from build123d import *

# Parameters (mm, degrees)
F0_W      = 15
F0_H      = 15
F1_DEPTH  = 25
F2_W      = 15
F2_H      = 15
F3_DEPTH  = 25
F4_DEPTH  = 10
F5_W      = 15
F5_H      = 15
F6_DEPTH  = 25
F7_W      = 5
F7_H      = 13
F8_DEPTH  = 25
F9_W      = 13
F9_H      = 5
F10_DEPTH = 20
F11_W     = 5
F11_H     = 13
F12_DEPTH = 25
F13_W     = 5
F13_H     = 5.5
F13_H_2   = 2.5
F14_DEPTH = 20


with BuildPart() as f1:
    # F0 (on Top) → F1 (new body)
    with BuildSketch(Plane.XY):
        with Locations((7.5, -7.5)):
            Rectangle(F0_W, F0_H)
    extrude(amount=F1_DEPTH)

    # F2 (on face) → F3 (join)
    with BuildSketch(Plane.XZ.offset(15)):
        with Locations((7.5, 7.5)):
            Rectangle(F2_W, F2_H)
    extrude(amount=F3_DEPTH)

    # F4 (add): a face of the model
    f4_faces = [f1.faces().sort_by_distance(p)[0] for p in [
        (7.5, -7.5, 25),
    ]]
    extrude(f4_faces, amount=F4_DEPTH)

    # F5 (on face) → F6 (join)
    with BuildSketch(Plane(origin=(0, 0, 0), x_dir=(0, -1, 0), z_dir=(-1, 0, 0))):
        with Locations((7.5, 7.5)):
            Rectangle(F5_W, F5_H)
    extrude(amount=F6_DEPTH)

    # F7 (on face) → F8 (cut, through all)
    with BuildSketch(Plane(origin=(-25, 0, 0), x_dir=(0, -1, 0), z_dir=(-1, 0, 0))):
        with Locations((10, 8.5)):
            Rectangle(F7_W, F7_H)
    extrude(amount=-F8_DEPTH, mode=Mode.SUBTRACT)

    # F9 (on face) → F10 (cut, through all)
    with BuildSketch(Plane.XY.offset(35)):
        with Locations((6.5, -10)):
            Rectangle(F9_W, F9_H)
    extrude(amount=-F10_DEPTH, mode=Mode.SUBTRACT)

    # F11 (on face) → F12 (cut, through all)
    with BuildSketch(Plane.XZ.offset(40)):
        with Locations((5, 8.5)):
            Rectangle(F11_W, F11_H)
    extrude(amount=-F12_DEPTH, mode=Mode.SUBTRACT)

    # F13 (on face) → F14 (cut, through all)
    with BuildSketch(Plane.XY.offset(35)):
        with Locations((5, -4.75)):
            Rectangle(F13_W, F13_H)
        with Locations((5, -13.75)):
            Rectangle(F13_W, F13_H_2)
    extrude(amount=-F14_DEPTH, mode=Mode.SUBTRACT)


solid = f1.part
Can you work these out from the model? Positions are in its coordinate system, mm. A direction names the side the tool comes from. Coordinates: 2 decimals unless noted, no trailing zeros. Write each loop counter-clockwise with the first axis right and the second up, starting at its lowest first coordinate (ties: lowest second). Pieces come first, ordered by that corner, then holes. Notation, with made-up numbers: M -30,-6 L -11,-6 A22 ccw -11,8 Z; hole C -36.5,27 d4. An arc over 180 degrees is marked long. Use one line per item in the form item = value.
Q1. For faces 1 (the flat face through (-12, -4, 15)), 2 (the flat face through (11, -27, 15)), 3 (the flat face through (-13, -10, 2)), 4 (the flat face through (5, -2, 25)), which set-ups out of +Z, -Z, +X, -X, +Y, -Y let a thin tool reach every point of the face, with its end or its side?
Model answer:
face_1 = +Z, -X, +Y, -Y
face_2 = +Z, +X, -X, -Y
face_3 = +Z, -X
face_4 = +Z, -Y
Q2. If we section it at B-B (x = 6): Write out the boundary of the cut face in (y, z).
Model answer:
outline = M -40,0 L 0,0 L 0,35 L -2,35 L -2,15 L -15,15 L -15,2 L -40,2 Z
Q3. If we section it at C-C (y = -18): Write out the boundary of the cut face in (x, z), then the cut area to 3 significant figures.
Model answer:
outline = M 0,0 L 15,0 L 15,15 L 7.5,15 L 7.5,2 L 2.5,2 L 2.5,15 L 0,15 Z
area = 160 mm^2
Q4. If we section it at D-D (z = 6.5): Write out the boundary of the cut face in (x, y), then the cut area to 3 significant figures.
Model answer:
outline = M -25,-15 L 0,-15 L 0,-40 L 2.5,-40 L 2.5,-15 L 7.5,-15 L 7.5,-40 L 15,-40 L 15,0 L -25,0 L -25,-7.5 L 0,-7.5 L 0,-12.5 L -25,-12.5 Z
area = 725 mm^2
Q5. For P1, Ø8, axis at x = -8, y = -3, coming from the +Z side; P2, Ø2, axis at y = -13.5, z = 25.5, coming from the -X side; P3, Ø6.5, axis at x = -7, z = 10.5, coming from the -Y side, each with a flat end and sliding along its axis, tell me the tip position at first contact or that it passes through.
Model answer:
P1 = 15
P2 = 0
P3 = -15
Q6. If we section it at A-A (z = 24.5): Write out the boundary of the cut face in (x, y), then the cut area to 3 significant figures.
Model answer:
outline = M 0,-15 L 2.5,-15 L 2.5,-12.5 L 0,-12.5 Z; M 0,-7.5 L 2.5,-7.5 L 2.5,-2 L 7.5,-2 L 7.5,-7.5 L 13,-7.5 L 13,-12.5 L 7.5,-12.5 L 7.5,-15 L 15,-15 L 15,0 L 0,0 Z
area = 120 mm^2
Q7. We'd pull the mould along X, two halves only. Please class faces 5 (the flat face through (7.5, -14, 25)), 6 (the flat face through (10, -7.5, 25)), 7 (the flat face through (0, -14, 25)): +X half, -X half, draft (parallel to the pull), parting line (faces both ways), or undercut.
Model answer:
face_5 = undercut
face_6 = draft
face_7 = -X half
Q8. I need wall thicknesses on line 1 along Y through (x, z) = (11, 26); line 2 along X through (y, z) = (-23, 8); line 3 along X through (y, z) = (-12, 16.5). Which ranges of each line are inside material? Lowest first, please. Write a range as from..to.
Model answer:
line_1 = -15..-12.5, -7.5..0
line_2 = 0..2.5, 7.5..15
line_3 = 13..15
